The drawing under review shows one solid part. Ordinate dimensions are in mm from its lowest x, y, z. Round coordinates to 2 decimals unless told otherwise and drop trailing zeros. Order: outer loops, then holes, each group sorted by start corner. A loop starts at its lowest first (then second) coordinate and runs counter-clockwise, first axis right, second up. Notation, with made-up numbers: M 29,-7.75 L 81,-7.75 A8 ccw 81,-0.75 Z; hole C -30.75,-15 d9. An arc over 180 degrees is marked long. Use a Markdown table: item, result.
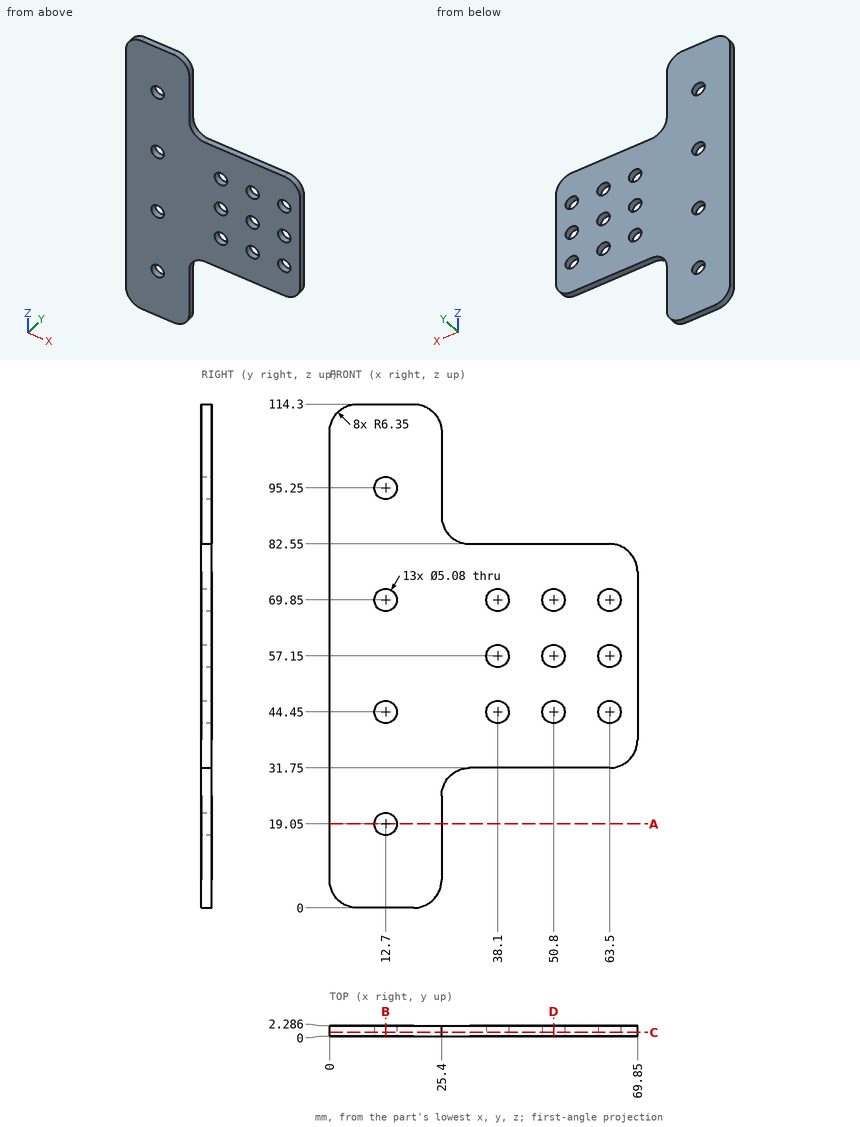
Q1. Wall thickness on line 1 along X through (y, z) = (1.1, 44.45); line 2 along Z through (x, y) = (50.5, 1); line 3 along X through (y, z) = (0.85, 95): over which ranges is each line inside the solid? List them lowest first. Write a range as [from, to].
Determined:
| item | result |
|---|---|
| line 1 | x = [0, 10.16], [15.24, 35.56], [40.64, 48.26], [53.34, 60.96], [66.04, 69.85] |
| line 2 | z = [31.75, 41.93], [46.97, 54.63], [59.67, 67.33], [72.37, 82.55] |
| line 3 | x = [0, 10.17], [15.23, 25.4] |
Q2. Clearance check with flat-ended pins moving along their axes: pin 1 (1.1 mm diameter, centred on x = 50, y = 1, fed in from -Z); pin 2 (0.7 mm diameter, centred on x = 47.5, y = 1, fed in from +Z). State where each tip first meets the part, or that it passes through.
Determined:
| item | result |
|---|---|
| pin 1 | stops at z = 31.75 |
| pin 2 | stops at z = 82.55 |
Q3. Add section C-C (y = 0.8). Give the number of separate pieces and of enclosed holes in the cut face, then the cut area to 3 significant figures.
Determined:
| item | result |
|---|---|
| separate pieces | 1 |
| enclosed holes | 13 |
| area | 4,860 mm^2 |
Q4. Add section A-A (z = 19.05). Write out the cut boundary in (x, y).
Determined:
| item | result |
|---|---|
| outline | M 0,0 L 10.16,0 L 10.16,2.29 L 0,2.29 Z; M 15.24,0 L 25.4,0 L 25.4,2.29 L 15.24,2.29 Z |
Q5. Add section D-D (x = 50.8). Write out the cut boundary in (y, z), then the cut area to 3 significant figures.
Determined:
| item | result |
|---|---|
| outline | M 0,31.75 L 2.29,31.75 L 2.29,41.91 L 0,41.91 Z; M 0,46.99 L 2.29,46.99 L 2.29,54.61 L 0,54.61 Z; M 0,59.69 L 2.29,59.69 L 2.29,67.31 L 0,67.31 Z; M 0,72.39 L 2.29,72.39 L 2.29,82.55 L 0,82.55 Z |
| area | 81.3 mm^2 |
Q6. Add section B-B (x = 12.7). Write out the cut boundary in (y, z).
Determined:
| item | result |
|---|---|
| outline | M 0,0 L 2.29,0 L 2.29,16.51 L 0,16.51 Z; M 0,21.59 L 2.29,21.59 L 2.29,41.91 L 0,41.91 Z; M 0,46.99 L 2.29,46.99 L 2.29,67.31 L 0,67.31 Z; M 0,72.39 L 2.29,72.39 L 2.29,92.71 L 0,92.71 Z; M 0,97.79 L 2.29,97.79 L 2.29,114.3 L 0,114.3 Z |
